```python
from build123d import *

# Parameters (mm, degrees)
SKETCH1_W           = 40
SKETCH1_H           = 40
BOSS_EXTRUDE1_DEPTH = 3
BOSS_EXTRUDE2_DEPTH = 40
SKETCH3_W           = 13.333333334
SKETCH3_H           = 6
CUT_EXTRUDE1_DEPTH  = 29.91366459


with BuildPart() as part:
    # Sketch1 → Boss-Extrude1 (new body)
    with BuildSketch(Plane(origin=(0, 0, 0), x_dir=(1, 0, 0), z_dir=(0, 1, 0))):
        Rectangle(SKETCH1_W, SKETCH1_H)
    extrude(amount=BOSS_EXTRUDE1_DEPTH)

    # Sketch2 → Boss-Extrude2 (add)
    with BuildSketch(Plane.XY.offset(20)):
        Polygon((-13.75, -6), (-6.25, -6), (-3.75, -3.5), (-5.946498308, -1.303501692), (-5.946498308, 0), (-14.053501692, 0), (-14.053501692, -1.303501692), (-16.25, -3.5), align=None)
    boss_extrude2 = extrude(amount=-BOSS_EXTRUDE2_DEPTH)

    # Sketch3 → Cut-Extrude1 (cut, through all)
    with BuildSketch(Plane(origin=(0, 0, 0), x_dir=(0, 0, -1), z_dir=(1, 0, 0))):
        with Locations((0, -3)):
            Rectangle(SKETCH3_W, SKETCH3_H)
    cut_extrude1 = extrude(amount=-CUT_EXTRUDE1_DEPTH, mode=Mode.SUBTRACT)

    # Mirror1: Boss-Extrude2, Cut-Extrude1 across plane
    add(boss_extrude2.mirror(Plane(origin=(0, 0, 0), x_dir=(0, 0, 1), z_dir=(1, 0, 0))))
    add(cut_extrude1.mirror(Plane(origin=(0, 0, 0), x_dir=(0, 0, 1), z_dir=(1, 0, 0))), mode=Mode.SUBTRACT)


solid = part.part
```
Geometry: final body of the model. Coordinates: model frame, mm. A direction names the side the tool comes from. Coordinates: 2 decimals unless noted, no trailing zeros. Order: outer loops, then holes, each group sorted by start corner. A loop starts at its lowest first (then second) coordinate and runs counter-clockwise, first axis right, second up. Notation, with made-up numbers: (33, 49) -> (49, 49) arc R18 cw to (49, 64) -> close; hole circle Ø8 at (35.25, 3.25). An arc over 180 degrees is marked (long way). Answer in a Markdown table with one row per item.
Item 1: Ray query, L1, parallel to Z at x = 10.5, y = -2.75; L2, parallel to X at y = -1, z = 14.5; L3, parallel to Y at x = 3, z = -9. Return the intervals inside material, ascending.
Return value:
| item | result |
|---|---|
| L1 | z = -20 to -6.67, 6.67 to 20 |
| L2 | x = -14.05 to -5.95, 5.95 to 14.05 |
| L3 | y = 0 to 3 |
Item 2: Section B-B on x = -4.5. Output: boundary loops of the cut face in (y, z), plus the area to 3 significant figures.
Return value:
| item | result |
|---|---|
| outline | (-4.25, -20) -> (-2.75, -20) -> (-2.75, -6.67) -> (-4.25, -6.67) -> close; (-4.25, 6.67) -> (-2.75, 6.67) -> (-2.75, 20) -> (-4.25, 20) -> close; (0, -20) -> (3, -20) -> (3, 20) -> (0, 20) -> close |
| area | 160 mm² |
Item 3: Section C-C on x = -11. Output: boundary loops of the cut face in (y, z), plus the area to 3 significant figures.
Return value:
| item | result |
|---|---|
| outline | (-6, -20) -> (3, -20) -> (3, 20) -> (-6, 20) -> (-6, 6.67) -> (0, 6.67) -> (0, -6.67) -> (-6, -6.67) -> close |
| area | 280 mm² |
Item 4: Section D-D on y = -5.5. Output: boundary loops of the cut face in (x, z).
Return value:
| item | result |
|---|---|
| outline | (-14.25, -20) -> (-5.75, -20) -> (-5.75, -6.67) -> (-14.25, -6.67) -> close; (-14.25, 6.67) -> (-5.75, 6.67) -> (-5.75, 20) -> (-14.25, 20) -> close; (5.75, -20) -> (14.25, -20) -> (14.25, -6.67) -> (5.75, -6.67) -> close; (5.75, 6.67) -> (14.25, 6.67) -> (14.25, 20) -> (5.75, 20) -> close |
Item 5: Section A-A on y = -3. Output: boundary loops of the cut face in (x, z).
Return value:
| item | result |
|---|---|
| outline | (-15.75, -20) -> (-4.25, -20) -> (-4.25, -6.67) -> (-15.75, -6.67) -> close; (-15.75, 6.67) -> (-4.25, 6.67) -> (-4.25, 20) -> (-15.75, 20) -> close; (4.25, -20) -> (15.75, -20) -> (15.75, -6.67) -> (4.25, -6.67) -> close; (4.25, 6.67) -> (15.75, 6.67) -> (15.75, 20) -> (4.25, 20) -> close |
Item 6: Contact query for flat-ended pins moving along their axis: P1, Ø20, axis at x = -1.5, z = -5, coming from the -Y side; P2, Ø1, axis at y = -1.5, z = 8, coming from the +X side; P3, Ø1.5, axis at y = -2.5, z = -7.5, coming from the -X side; P4, Ø1, axis at y = -1, z = 11, coming from the +X side. Output: stop coordinate, or through.
Return value:
| item | result |
|---|---|
| P1 | stops at y = -6 |
| P2 | stops at x = 14.75 |
| P3 | stops at x = -16 |
| P4 | stops at x = 14.25 |
Item 7: Access query for faces 1 (the flat face through (-5.02, -4.77, 13.43)), 2 (the flat face through (-10, -3, -6.667)), 3 (the flat face through (5.946, -1, 13)). Directions: +Z, -Z, +X, -X, +Y, -Y. A direction counts if a zero-diameter tool reaches every point of the face in a straight line with its end or side. Return the directions, or none.
Return value:
| item | result |
|---|---|
| face 1 | +Z, -Z, -Y |
| face 2 | +X, -X, -Y |
| face 3 | +Z, -Z |
Item 8: Draft query along X for faces 4 (the flat face through (-4.83, -2.42, 13.43)), 5 (the flat face through (-14.054, -1, -13)), 6 (the flat face through (4.83, -2.42, -13.24)), 7 (the flat face through (10, -3, 6.667)). Return one class per face: released by +X, released by -X, zero draft, split by the parting line, or undercut.
Return value:
| item | result |
|---|---|
| face 4 | undercut |
| face 5 | released by -X |
| face 6 | undercut |
| face 7 | zero draft |
